The listing builds one solid part. Answer for the finished solid, in the listing's coordinates (mm). Coordinates: 2 decimals unless noted, no trailing zeros. Write each loop counter-clockwise with the first axis right and the second up, starting at its lowest first coordinate (ties: lowest second). Pieces come first, ordered by that corner, then holes. Notation, with made-up numbers: M 9,-29 L 39,-29 A28 cw 39,4 Z; hole C 82.25,16.25 d6. An arc over 180 degrees is marked long. Answer as a JSON object with one key per item and string values. Group by question number.
from build123d import *

# Parameters (mm, degrees)
F1_DEPTH  = 18
F3_DEPTH  = 5
F5_DEPTH  = 7
F6_R      = 12.5
F6_R_2    = 3.5
F7_DEPTH  = 25
F8_R      = 10
F8_R_2    = 3.5
F9_DEPTH  = 1
F10_R     = 3.902724
F11_DEPTH = 25


with BuildPart() as f1:
    # F0 (on Top) → F1 (new body)
    with BuildSketch(Plane.XY):
        with BuildLine():
            Line((600, 60), (600, 0))
            Line((600, 0), (1200, 0))
            Line((1200, 0), (1200, 350))
            Line((1200, 350), (0, 350))
            Line((0, 350), (0, 90))
            Line((0, 90), (570, 90))
            ThreePointArc((570, 90), (591.213203, 81.213203), (600, 60))
        make_face()
    extrude(amount=F1_DEPTH)

    # F2 (on face) → F3 (join)
    with BuildSketch(Plane(origin=(0, 0, 0), x_dir=(1, 0, 0), z_dir=(0, 0, -1))):
        with BuildLine():
            Line((600, 0), (600, -60))
            ThreePointArc((600, -60), (591.213203, -81.213203), (570, -90))
            Line((570, -90), (0, -90))
            Line((0, -90), (0, -350))
            Line((0, -350), (1200, -350))
            Line((1200, -350), (1200, 0))
            Line((1200, 0), (600, 0))
        make_face()
        with BuildLine():
            Line((369, -105), (555, -105))
            ThreePointArc((555, -105), (558.535534, -106.464466), (560, -110))
            Line((560, -110), (560, -150))
            ThreePointArc((560, -150), (558.535534, -153.535534), (555, -155))
            Line((555, -155), (369, -155))
            ThreePointArc((369, -155), (365.464466, -153.535534), (364, -150))
            Line((364, -150), (364, -110))
            ThreePointArc((364, -110), (365.464466, -106.464466), (369, -105))
        make_face(mode=Mode.SUBTRACT)
    extrude(amount=F3_DEPTH)

    # F4 (on face) → F5 (cut)
    with BuildSketch(Plane(origin=(0, 0, -5), x_dir=(1, 0, 0), z_dir=(0, 0, -1))):
        with BuildLine():
            Line((125, -90), (0, -90))
            Line((0, -90), (0, -114.8))
            Line((0, -114.8), (120, -114.8))
            ThreePointArc((120, -114.8), (123.535534, -113.335534), (125, -109.8))
            Line((125, -109.8), (125, -90))
        make_face()
    extrude(amount=-F5_DEPTH, mode=Mode.SUBTRACT)

    # F6 (on face) → F7 (cut)
    with BuildSketch(Plane(origin=(0, 0, 0), x_dir=(1, 0, 0), z_dir=(0, 0, -1))):
        with Locations((525, -130)):
            Circle(F6_R)
        with Locations((399, -130)):
            Circle(F6_R)
        with Locations((371, -112)):
            Circle(F6_R_2)
        with Locations((427, -112)):
            Circle(F6_R_2)
        with Locations((371, -148)):
            Circle(F6_R_2)
        with Locations((427, -148)):
            Circle(F6_R_2)
        with Locations((497, -148)):
            Circle(F6_R_2)
        with Locations((497, -112)):
            Circle(F6_R_2)
        with Locations((553, -112)):
            Circle(F6_R_2)
        with Locations((553, -148)):
            Circle(F6_R_2)
    extrude(amount=-F7_DEPTH, mode=Mode.SUBTRACT)

    # F8 (on face) → F9 (cut)
    with BuildSketch(Plane.XY.offset(18)):
        with Locations((371, 148)):
            Circle(F8_R)
        with Locations((371, 148)):
            Circle(F8_R_2, mode=Mode.SUBTRACT)
        with Locations((427, 148)):
            Circle(F8_R)
        with Locations((427, 148)):
            Circle(F8_R_2, mode=Mode.SUBTRACT)
        with Locations((497, 148)):
            Circle(F8_R)
        with Locations((497, 148)):
            Circle(F8_R_2, mode=Mode.SUBTRACT)
        with Locations((553, 148)):
            Circle(F8_R)
        with Locations((553, 148)):
            Circle(F8_R_2, mode=Mode.SUBTRACT)
        with Locations((553, 112)):
            Circle(F8_R)
        with Locations((553, 112)):
            Circle(F8_R_2, mode=Mode.SUBTRACT)
        with Locations((497, 112)):
            Circle(F8_R)
        with Locations((497, 112)):
            Circle(F8_R_2, mode=Mode.SUBTRACT)
        with Locations((427, 112)):
            Circle(F8_R)
        with Locations((427, 112)):
            Circle(F8_R_2, mode=Mode.SUBTRACT)
        with Locations((371, 112)):
            Circle(F8_R)
        with Locations((371, 112)):
            Circle(F8_R_2, mode=Mode.SUBTRACT)
    extrude(amount=-F9_DEPTH, mode=Mode.SUBTRACT)

    # F10 (on face) → F11 (cut)
    with BuildSketch(Plane(origin=(0, 0, 2), x_dir=(1, 0, 0), z_dir=(0, 0, -1))):
        with Locations((111.9, -103.2)):
            Circle(F10_R)
        with Locations((91.9, -103.2)):
            Circle(F10_R)
        with Locations((71.9, -103.2)):
            Circle(F10_R)
        with Locations((51.9, -103.2)):
            Circle(F10_R)
        with Locations((31.9, -103.2)):
            Circle(F10_R)
    extrude(amount=-F11_DEPTH, mode=Mode.SUBTRACT)


solid = f1.part
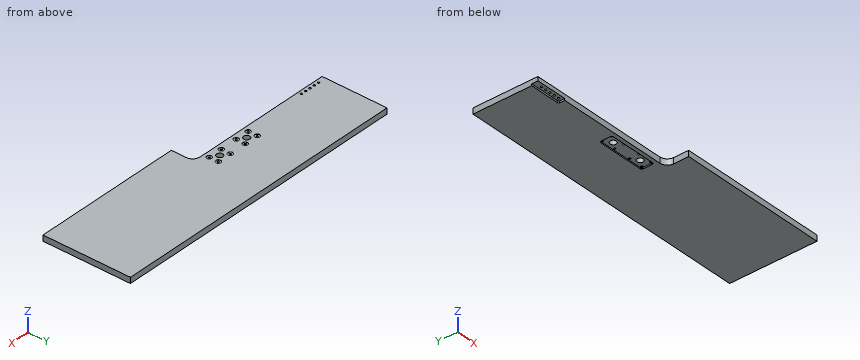
Item 1: Consider L1, parallel to Y at x = 371, z = 17.35; L2, parallel to X at y = 103.2, z = 13.5; L3, parallel to Y at x = 111.9, z = 13. Determine where each line is inside the solid, lowest interval first. Write a range as from..to.
Item 2: A cutting plane is placed at B-B, the plane x = 274. Write down the section's boundary in (y, z).
Item 3: A cutting plane is placed at A-A, the plane z = 10.75. State how many separate pieces and enclosed holes the cut face has, and give its area (3 significant figures).
Answer:
{
 "1": {"L1": "90..102, 122..138, 158..350", "L2": "0..28, 35.8..48, 55.8..68, 75.8..88, 95.8..108, 115.8..1200", "L3": "90..99.3, 107.1..350"},
 "2": {"outline": "M 90,-5 L 350,-5 L 350,18 L 90,18 Z"},
 "3": {"separate pieces": "1", "enclosed holes": "15", "area": "365,000 mm2"}
}
